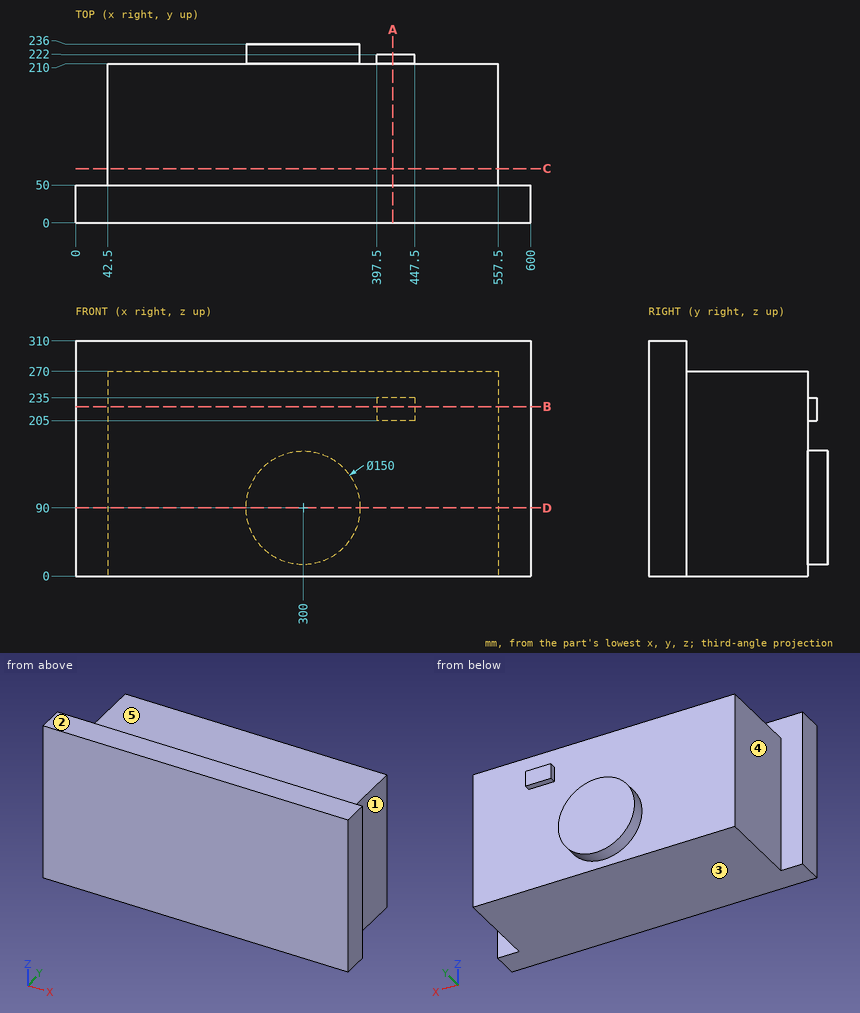
Design review of the part shown in the three views and the two pictorial views. Dimensions are in mm from the part's minimum x, y and z. A direction names the side the tool comes from. Give positions to 0.01 mm unless a question says otherwise; leave off trailing zeros. Order: outer loops, then holes, each group sorted by start corner. A loop starts at its lowest first (then second) coordinate and runs counter-clockwise, first axis right, second up. Notation, with made-up numbers: (-9, 5) -> (6, 5) arc R11 ccw to (6, 18) -> close; hole circle Ø7 at (-18.5, 68.25). An arc over 180 degrees is marked (long way). Write each question's results on one line, items separated by ' | '. Start each with the question number.
Q1. Machinability: for the marked faces 1, 2, 3, 4 and 5, which of the approach directions +Z, -Z, +X, -X, +Y, -Y give a long, thin tool a straight path to every point of the face, cutting with its end or side? Answer none if there is none.
Q2. For pin 1 (6 mm diameter, centred on y = 214, z = 214, fed in from +X); pin 2 (8 mm diameter, centred on y = 61, z = 259, fed in from +X); pin 3 (1.5 mm diameter, centred on x = 382, z = 183, fed in from +Y), all flat-tipped, find the tip position at first contact; note any pin that passes through.
Q3. Add section B-B on z = 223.5. Give the boundary of the cut face in (x, y), and give its area (3 significant figures).
Q4. Add section C-C on y = 71.5. Give the boundary of the cut face in (x, z).
Q5. Add section A-A on x = 418.5. Give the boundary of the cut face in (y, z).
Q6. Wall thickness on L1, parallel to Z at x = 142.5, y = 165.5; L2, parallel to X at y = 55, z = 222; L3, parallel to Y at x = 450.5, z = 63: over which ranges is each line inside the solid? List them lowest first. Write a range as from..to.
Q7. Add section D-D on z = 90. Give the boundary of the cut face in (x, y), and give its area (3 significant figures).
Found:
1) face 1: +Z, -Z, +X, +Y | face 2: +Z, +X, -X, +Y, -Y | face 3: -Z, +X, -X, +Y, -Y | face 4: +Z, -Z, -X, +Y | face 5: +Z, +X, -X, +Y
2) pin 1: stops at x = 447.5 | pin 2: stops at x = 557.5 | pin 3: stops at y = 210
3) outline: (0, 0) -> (600, 0) -> (600, 50) -> (557.5, 50) -> (557.5, 210) -> (447.5, 210) -> (447.5, 222) -> (397.5, 222) -> (397.5, 210) -> (42.5, 210) -> (42.5, 50) -> (0, 50) -> close | area: 113,000 mm2
4) outline: (42.5, 0) -> (557.5, 0) -> (557.5, 270) -> (42.5, 270) -> close
5) outline: (0, 0) -> (210, 0) -> (210, 205) -> (222, 205) -> (222, 235) -> (210, 235) -> (210, 270) -> (50, 270) -> (50, 310) -> (0, 310) -> close
6) L1: z = 0..270 | L2: x = 42.5..557.5 | L3: y = 0..210
7) outline: (0, 0) -> (600, 0) -> (600, 50) -> (557.5, 50) -> (557.5, 210) -> (375, 210) -> (375, 236) -> (225, 236) -> (225, 210) -> (42.5, 210) -> (42.5, 50) -> (0, 50) -> close | area: 116,000 mm2
